```python
from build123d import *

# Parameters (mm, degrees)
BOSS_EXTRUDE1_DEPTH     = 5.715
CUT_EXTRUDE1_DEPTH      = 6.715
SKETCH4_R               = 4.6355
CUT_EXTRUDE2_DEPTH      = 1
CUT_EXTRUDE2_DEPTH_BACK = 6.715
SKETCH5_W               = 254
SKETCH5_H               = 5.08
CUT_EXTRUDE3_DEPTH      = 6.715


with BuildPart() as part:
    # Sketch1 → Boss-Extrude1 (new body)
    with BuildSketch(Plane.XY):
        Polygon((6.35, -63.5), (127, -63.5), (127, -5.715), (132.715, -5.715), (132.715, 6.985), (127, 6.985), (127, 63.5), (-127, 63.5), (-127, 6.985), (-132.715, 6.985), (-132.715, -5.715), (-127, -5.715), (-127, -63.5), (-6.35, -63.5), (-6.35, -69.215), (6.35, -69.215), align=None)
    extrude(amount=BOSS_EXTRUDE1_DEPTH)

    # Sketch2 → Cut-Extrude1 (cut, through all)
    with BuildSketch(Plane.XY.offset(5.715)):
        with BuildLine():
            Line((76.2, -3.175), (-76.2, -3.175))
            ThreePointArc((-76.2, -3.175), (-79.375, 0), (-76.2, 3.175))
            Line((-76.2, 3.175), (76.2, 3.175))
            ThreePointArc((76.2, 3.175), (79.375, 0), (76.2, -3.175))
        make_face()
    extrude(amount=-CUT_EXTRUDE1_DEPTH, mode=Mode.SUBTRACT)

    # Sketch4 → Cut-Extrude2 (cut, two sides)
    with BuildSketch(Plane.XY.offset(5.715)) as cut_extrude2_sk:
        with Locations((0, -50.8)):
            Circle(SKETCH4_R)
    extrude(amount=CUT_EXTRUDE2_DEPTH, mode=Mode.SUBTRACT)
    extrude(cut_extrude2_sk.sketch, amount=-CUT_EXTRUDE2_DEPTH_BACK, mode=Mode.SUBTRACT)

    # Sketch5 → Cut-Extrude3 (cut, through all)
    with BuildSketch(Plane.XY.offset(5.715)):
        with Locations((0, 60.96)):
            Rectangle(SKETCH5_W, SKETCH5_H)
    extrude(amount=-CUT_EXTRUDE3_DEPTH, mode=Mode.SUBTRACT)


solid = part.part
```
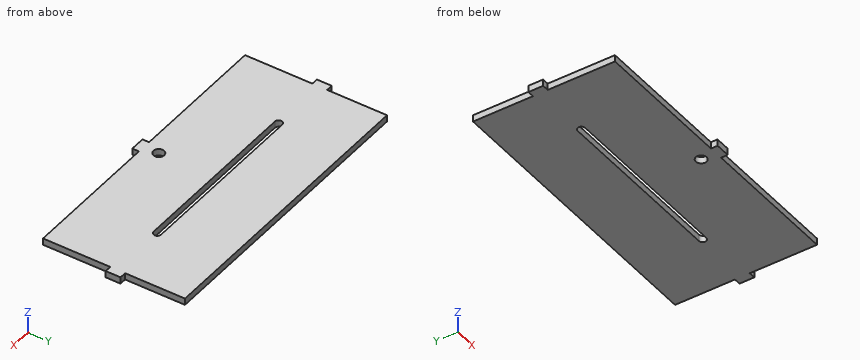
Geometry: final body of the model. Coordinates: model frame, mm. Round coordinates to 2 decimals unless told otherwise and drop trailing zeros. Order: outer loops, then holes, each group sorted by start corner. A loop starts at its lowest first (then second) coordinate and runs counter-clockwise, first axis right, second up. Notation, with made-up numbers: (6, -12.5) -> (39, -12.5) arc R8 cw to (39, -8.5) -> close; hole circle Ø4 at (65, 44.5). An arc over 180 degrees is marked (long way). Use one line per item in the form item = value. Start each with the question number.
1. Pin query (flat end, axial travel): pin 1 Ø1.7 at (y, z) = (39.5, 2) entering from -X; pin 2 Ø1.7 at (x, z) = (130, 1.5) entering from +Y (3 decimals); pin 3 Ø8.5 at (x, y) = (0, -50.8) entering from +Z; pin 4 Ø1.7 at (x, z) = (-131, 4) entering from -Y (3 decimals). Return the tip coordinate at first contact, or that it passes through.
2. Cut plane B-B (z = 3.4). Count the separate pieces of the cut face and the enclosed holes in it, then the cut area to 3 significant figures.
3. Cut plane C-C (y = 0). Return the cut outline in (x, z) (3 decimals).
4. Line query: probe 1 along Y at (x, z) = (0, 1.35) (1 decimal); probe 2 along Y at (x, z) = (19, 5.2) (3 decimals); probe 3 along Y at (x, z) = (99.5, 2.55). Output: solid intervals per line, ascending.
5. Cut plane D-D (y = 33). Return the cut outline in (x, z) (3 decimals).
6. Cut plane A-A (y = -50.8). Return the cut outline in (x, z) (1 decimal).
Solution:
q1.pin_1 = -127
q1.pin_2 = 6.985
q1.pin_3 = through
q1.pin_4 = -5.715
q2.separate_pieces = 1
q2.enclosed_holes = 2
q2.area = 30,100 mm^2
q3.outline = (-132.715, 0) -> (-79.375, 0) -> (-79.375, 5.715) -> (-132.715, 5.715) -> close; (79.375, 0) -> (132.715, 0) -> (132.715, 5.715) -> (79.375, 5.715) -> close
q4.probe_1 = -69.2 to -55.4, -46.2 to -3.2, 3.2 to 58.4
q4.probe_2 = -63.5 to -3.175, 3.175 to 58.42
q4.probe_3 = -63.5 to 58.42
q5.outline = (-127, 0) -> (127, 0) -> (127, 5.715) -> (-127, 5.715) -> close
q6.outline = (-127, 0) -> (-4.6, 0) -> (-4.6, 5.7) -> (-127, 5.7) -> close; (4.6, 0) -> (127, 0) -> (127, 5.7) -> (4.6, 5.7) -> close
